Work out the finished part from the listing and answer in its coordinate system (mm). A direction names the side the tool comes from. Coordinates: 2 decimals unless noted, no trailing zeros. Loops run counter-clockwise (first coordinate to the right, second up) from the corner with the lowest first, then second, coordinate; pieces in that order, holes last. Notation, with made-up numbers: (49.5, 64.25) - (77.5, 64.25) arc R11 cw to (77.5, 78.25) - close; hole circle Ø4 at (-26.5, -13.75). An arc over 180 degrees is marked (long way). Write each question's results on one line, items separated by ' | '. Start each with the question number.
1. Determine the mould class of faces 1 (the cylindrical face through (5.43, -4.4, -7.6)), 2 (the flat face through (5.5, 4.6, 0)), 3 (the cylindrical face through (5.4, 4.43, -7.6)) for opening direction Y: released by +Y, released by -Y, zero draft, split by the parting line, or undercut.
2. This flat-tipped pin is pushed along its axis until it touches: P1, Ø1, axis at x = -4.5, z = -7, coming from the -Y side. Where does it stop, or does it pass through?
3. A cutting plane is placed at C-C on x = 3.25. Determine the outline of the cut face in (y, z), then the cut area to 3 significant figures.
4. Find the intervals of material crossed by line 1 along Z through (x, y) = (-3.5, -0.25); line 2 along X through (y, z) = (-3.5, -2); line 3 along Y through (x, z) = (-0.5, 13), in increasing order. Write a range as [from, to].
5. A cutting plane is placed at A-A on x = 0. Determine the outline of the cut face in (y, z).
6. A cutting plane is placed at B-B on y = 0. Determine the outline of the cut face in (x, z).
7. Which of the six approach directions +Z, -Z, +X, -X, +Y, -Y give full straight-line access (tool end or side, diameter ignored) to faces 4 (the cylindrical face through (-5.4, -4.43, -7.6)), 5 (the cylindrical face through (-1.5, -0.07, 13.93)), 6 (the flat face through (5.6, -4.6, 0))?
Autodesk Fusion 360 part; units mm, degrees
sketch "草图1" plane through (0, 0, 0) normal (0, 0, 1) x (1, 0, 0)
  line L0 (6, -5) -> (-6, -5)
  line L1 (-6, -5) -> (-6, 5)
  line L2 (-6, 5) -> (6, 5)
  line L3 (6, 5) -> (6, -5)
  line L4 (6, -5) -> (-6, 5) construction
  line L5 (-6, -5) -> (6, 5) construction
  circle A0 centre (0, 0) radius 1.5
  dimension "d1" = 12
  dimension "d2" = 10
  dimension "d3" = 3
extrude "拉伸1" add sketch "草图1" along normal blind 9 contours L0 L1 L2 L3 | A0 makes body 1
extrude "拉伸2" add sketch "草图1" against normal blind 15 separate body contours L0 L1 L2 L3 | A0 makes body 2
fillet "圆角1" radius 2 4 edges at (6, 5, -7.5) (-6, 5, -7.5) (6, -5, -7.5) (-6, -5, -7.5) on bodies 2
extrude "拉伸3" add sketch "草图1" along normal blind 19 contours A0 bodies 1 2
Values:
1) face 1: released by -Y | face 2: zero draft | face 3: released by +Y
2) P1: y = -5
3) outline: (-5, -15) - (5, -15) - (5, 9) - (-5, 9) - close | area: 240 mm^2
4) line 1: [-15, 9] | line 2: [-5.94, 5.94] | line 3: [-1.41, 1.41]
5) outline: (-5, -15) - (5, -15) - (5, 9) - (1.5, 9) - (1.5, 19) - (-1.5, 19) - (-1.5, 9) - (-5, 9) - close
6) outline: (-6, -15) - (6, -15) - (6, 9) - (1.5, 9) - (1.5, 19) - (-1.5, 19) - (-1.5, 9) - (-6, 9) - close
7) face 4: -Z, -X, -Y | face 5: +Z | face 6: -Z, +X, -Y
